Could you check a few things on this drawing? It's one solid part, dimensions in mm from its lowest x, y, z. A direction names the side the tool comes from. Give positions to 0.01 mm unless a question says otherwise; leave off trailing zeros. Loops run counter-clockwise (first coordinate to the right, second up) from the corner with the lowest first, then second, coordinate; pieces in that order, holes last. Notation, with made-up numbers: M 58.5,-13.5 L 65.5,-13.5 A35 ccw 65.5,25.5 Z; hole C -27,12.5 d4. An arc over 180 degrees is marked long. Answer as a JSON object with one key per item and string values.
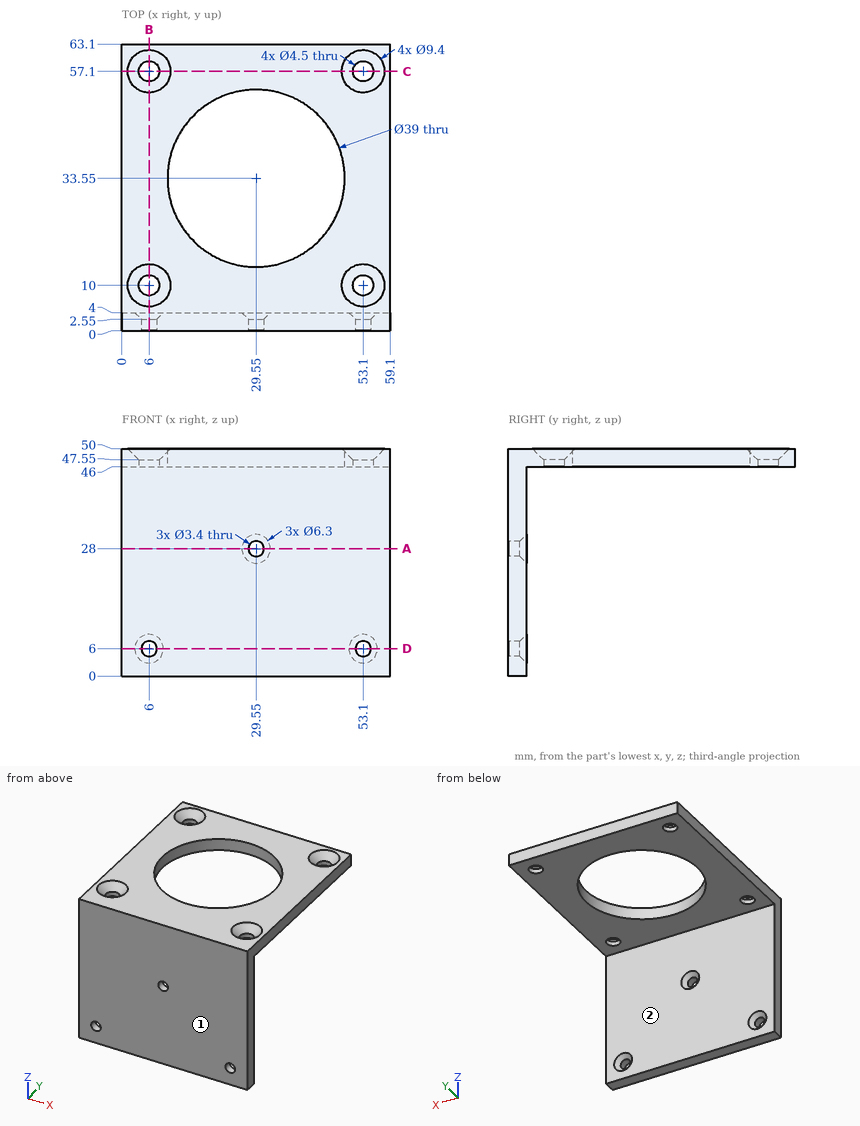
1) Suppose I cut it at B-B, the plane x = 6. Write out the boundary of the cut face in (y, z), and give its area (3 significant figures).
Answer list:
{"outline": "M 0,0 L 4,0 L 4,2.85 L 2.55,4.3 L 0,4.3 Z; M 0,7.7 L 2.55,7.7 L 4,9.15 L 4,46 L 7.75,46 L 7.75,47.55 L 5.3,50 L 0,50 Z; M 12.25,46 L 54.85,46 L 54.85,47.55 L 52.4,50 L 14.7,50 L 12.25,47.55 Z; M 59.35,46 L 63.1,46 L 63.1,50 L 61.8,50 L 59.35,47.55 Z", "area": "373 mm^2"}
2) Suppose I cut it at C-C, the plane y = 57.1. Write out the boundary of the cut face in (x, z).
Answer list:
{"outline": "M 0,46 L 3.75,46 L 3.75,47.55 L 1.3,50 L 0,50 Z; M 8.25,46 L 50.85,46 L 50.85,47.55 L 48.4,50 L 10.7,50 L 8.25,47.55 Z; M 55.35,46 L 59.1,46 L 59.1,50 L 57.8,50 L 55.35,47.55 Z"}
3) Suppose I cut it at A-A, the plane z = 28. Write out the boundary of the cut face in (x, y), and give its area (3 significant figures).
Answer list:
{"outline": "M 0,0 L 27.85,0 L 27.85,2.55 L 26.4,4 L 0,4 Z; M 31.25,0 L 59.1,0 L 59.1,4 L 32.7,4 L 31.25,2.55 Z", "area": "221 mm^2"}
4) Please list where these lines run through material, in increasing order: line 1 along X through (y, z) = (57.1, 47.15); line 2 along Y through (x, z) = (53, 47); line 3 along Y through (x, z) = (29, 48). Write a range as from..to.
Answer list:
{"line 1": "0..3.75, 8.25..50.85, 55.35..59.1", "line 2": "0..7.75, 12.25..54.85, 59.35..63.1", "line 3": "0..14.06, 53.04..63.1"}
5) Will these pins go through, and if not, where does the flat tip stop? pin 1 Ø3 at (x, z) = (45, 44) entering from +Y; pin 2 Ø6 at (x, y) = (6, 10) entering from -Z.
Answer list:
{"pin 1": "y = 4", "pin 2": "z = 46"}
6) Suppose I cut it at D-D, the plane z = 6. Write out the boundary of the cut face in (x, y).
Answer list:
{"outline": "M 0,0 L 4.3,0 L 4.3,2.55 L 2.85,4 L 0,4 Z; M 7.7,0 L 51.4,0 L 51.4,2.55 L 49.95,4 L 9.15,4 L 7.7,2.55 Z; M 54.8,0 L 59.1,0 L 59.1,4 L 56.25,4 L 54.8,2.55 Z"}
7) For the marked faces 1 and 2, which set-ups out of +Z, -Z, +X, -X, +Y, -Y let a thin tool reach every point of the face, with its end or its side?
Answer list:
{"face 1": "+Z, -Z, +X, -X, -Y", "face 2": "-Z, +X, -X, +Y"}
